For this review, take the finished solid that the model builds, in its own axes (mm). A direction names the side the tool comes from. Coordinates: 2 decimals unless noted, no trailing zeros. Write each loop counter-clockwise with the first axis right and the second up, starting at its lowest first coordinate (ties: lowest second). Pieces come first, ordered by that corner, then holes.
```python
from build123d import *

# Parameters (mm, degrees)
SKETCH004_W     = 39.5
SKETCH004_H     = 37
SKETCH004_W_2   = 25.5
SKETCH004_H_2   = 29
PAD002_DEPTH    = 20
SKETCH005_R     = 3.425
HOLE003_DEPTH   = 5
HOLE003_TIPS_R  = 3.425
SKETCH006_R     = 4.25
HOLE004_DEPTH   = 15
HOLE004_TIPS_R  = 4.25
POCKET_DEPTH    = 6
SKETCH008_W     = 8.5
SKETCH008_H     = 10
POCKET001_DEPTH = 15
FILLET003_R     = 3


with BuildPart() as part:
    # Sketch004 → Pad002 (new body)
    with BuildSketch(Plane.XY):
        with Locations((19.75, 18.5)):
            Rectangle(SKETCH004_W, SKETCH004_H)
        with Locations((16.75, 18.5)):
            Rectangle(SKETCH004_W_2, SKETCH004_H_2, mode=Mode.SUBTRACT)
    extrude(amount=PAD002_DEPTH)

    # Sketch005 (on Face4 of Pad002) → Hole003 (cut)
    with BuildSketch(Plane(origin=(0, 0, 0), x_dir=(0, -1, 0), z_dir=(-1, 0, 0))):
        with Locations((-18.5, 10)):
            Circle(SKETCH005_R)
    extrude(amount=-HOLE003_DEPTH, mode=Mode.SUBTRACT)

    # Hole003 tips → Hole003 tip 1 section 0
    with BuildSketch(Plane(origin=(5, 0, 0), x_dir=(0, -1, 0), z_dir=(-1, 0, 0)), mode=Mode.PRIVATE) as hole003_tip_1_s0:
        with Locations((-18.5, 10)):
            Circle(HOLE003_TIPS_R)
    loft([hole003_tip_1_s0.sketch, Vertex(7.057948, 18.5, 10)], mode=Mode.SUBTRACT)

    # Sketch006 (on Face3 of Hole003) → Hole004 (cut)
    with BuildSketch(Plane.YZ.offset(39.5)):
        with Locations((18.5, 10)):
            Circle(SKETCH006_R)
    extrude(amount=-HOLE004_DEPTH, mode=Mode.SUBTRACT)

    # Hole004 tips → Hole004 tip 1 section 0
    with BuildSketch(Plane.YZ.offset(24.5), mode=Mode.PRIVATE) as hole004_tip_1_s0:
        with Locations((18.5, 10)):
            Circle(HOLE004_TIPS_R)
    loft([hole004_tip_1_s0.sketch, Vertex(21.946342, 18.5, 10)], mode=Mode.SUBTRACT)

    # Sketch007 (on Face10 of Hole004) → Pocket (cut)
    with BuildSketch(Plane(origin=(29.5, 0, 0), x_dir=(0, -1, 0), z_dir=(-1, 0, 0))):
        Polygon((-11.75, 13.897114), (-18.5, 17.794229), (-25.25, 13.897114), (-25.25, 6.102886), (-18.5, 2.205771), (-11.75, 6.102886), align=None)
    extrude(amount=-POCKET_DEPTH, mode=Mode.SUBTRACT)

    # Sketch008 (on Face3 of Pocket) → Pocket001 (cut)
    with BuildSketch(Plane.YZ.offset(39.5)):
        with Locations((18.5, 15)):
            Rectangle(SKETCH008_W, SKETCH008_H)
    extrude(amount=-POCKET001_DEPTH, mode=Mode.SUBTRACT)

    # Fillet003
    fillet003_edges = [part.edges().sort_by_distance(p)[0] for p in [
        (0, 0, 10),
        (39.5, 0, 10),
        (0, 37, 10),
        (39.5, 37, 10),
    ]]
    fillet(fillet003_edges, radius=FILLET003_R)


solid = part.part
```
Q1. Add section C-C (z = 17.5). State the section outline as (x, y) points.
Ans:
outline: (0, 3) arc R3 ccw to (3, 0) - (36.5, 0) arc R3 ccw to (39.5, 3) - (39.5, 14.25) - (29.5, 14.25) - (29.5, 4) - (4, 4) - (4, 33) - (29.5, 33) - (29.5, 22.75) - (39.5, 22.75) - (39.5, 34) arc R3 ccw to (36.5, 37) - (3, 37) arc R3 ccw to (0, 34) - close
Q2. Tool access review of faces 1 (the flat face through (32, 11.75, 10)), 2 (the flat face through (17, 4, 10)), 3 (the flat face through (36, 14.25, 16)): name each direction out of +Z, -Z, +X, -X, +Y, -Y from which nothing blocks a thin tool from reaching the whole face with its end or side.
Ans:
face 1: none
face 2: +Z, -Z
face 3: +Z, +X
Q3. For probe 1 along X at (y, z) = (29, 18.5); probe 2 along Y at (x, z) = (27, 3.75); probe 3 along Y at (x, z) = (35, 18), list the stretches that pass through material, from the lowest coordinate up.
Ans:
probe 1: x = 0 to 4, 29.5 to 39.5
probe 2: y = 0 to 4, 33 to 37
probe 3: y = 0 to 14.25, 22.75 to 37
Q4. Clearance check with a flat-ended pin moving along its axis: pin 1 Ø10 at (x, y) = (9.5, 26) entering from +Z. State where the tip first meets the part, or that it passes through.
Ans:
pin 1: passes through
Q5. Add section A-A (x = 27). State the section outline as (y, z) points, then the cut area to 3 significant figures.
Ans:
outline: (0, 0) - (4, 0) - (4, 20) - (0, 20) - close; (33, 0) - (37, 0) - (37, 20) - (33, 20) - close
area: 160 mm2
Q6. Add section B-B (y = 5). State the section outline as (x, z) points, then the cut area to 3 significant figures.
Ans:
outline: (0, 0) - (4, 0) - (4, 20) - (0, 20) - close; (29.5, 0) - (39.5, 0) - (39.5, 20) - (29.5, 20) - close
area: 280 mm2
Q7. Draft analysis for pull direction Z (two halves, no side actions). For faces 4 (the flat face through (4, 15, 8)), 5 (the flat face through (35.5, 20.1, 5.9)), 6 (the flat face through (33, 19, 0)), state which applies: +Z half, -Z half, draft (parallel to the pull), parting line (faces both ways), or undercut.
Ans:
face 4: draft
face 5: undercut
face 6: -Z half
Q8. Add section D-D (y = 16). State the section outline as (x, z) points.
Ans:
outline: (0, 0) - (4, 0) - (4, 7.66) - (0, 7.66) - close; (0, 12.34) - (4, 12.34) - (4, 20) - (0, 20) - close; (29.5, 0) - (39.5, 0) - (39.5, 6.56) - (35.5, 6.56) - (35.5, 3.65) - (29.5, 3.65) - close
